```python
from build123d import *

# Parameters (mm, degrees)
AUFSATZ_LINEAR_AUSTRAGEN1_DEPTH      = 25
AUFSATZ_LINEAR_AUSTRAGEN1_DEPTH_BACK = 12.5
SKIZZE1_W                            = 33
SKIZZE1_H                            = 15
SKIZZE2_W                            = 28
SKIZZE2_H                            = 12
SCHNITT_LINEAR_AUSTRAGEN1_DEPTH      = 42.650330131
M3_GEWINDEBOHRUNG1_D                 = 2.5
M4_GEWINDEBOHRUNG1_D                 = 3.3
SCHNITT_LINEAR_AUSTRAGEN2_DEPTH      = 34.5


with BuildPart() as part:
    # Skizze1 → Aufsatz-Linear austragen1 (new, two sides: drawn at the far end of the back side and taken through both)
    with BuildSketch(Plane.XY.offset(-AUFSATZ_LINEAR_AUSTRAGEN1_DEPTH_BACK)):
        Rectangle(SKIZZE1_W, SKIZZE1_H)
    extrude(amount=AUFSATZ_LINEAR_AUSTRAGEN1_DEPTH + AUFSATZ_LINEAR_AUSTRAGEN1_DEPTH_BACK)

    # Skizze2 → Schnitt-Linear austragen1 (cut, through all)
    with BuildSketch(Plane.XY.offset(25)):
        with Locations((-2.5, -1.5)):
            Rectangle(SKIZZE2_W, SKIZZE2_H)
    extrude(amount=-SCHNITT_LINEAR_AUSTRAGEN1_DEPTH, mode=Mode.SUBTRACT)

    # M3 Gewindebohrung1 (through all)
    with Locations(Plane(origin=(0, 7.5, 0), x_dir=(1, 0, 0), z_dir=(0, 1, 0))):
        with Locations((-9.5, 0)):
            Hole(M3_GEWINDEBOHRUNG1_D / 2)

    # M4 Gewindebohrung1 (through all)
    with Locations(Plane(origin=(16.5, 0, 0), x_dir=(0, 0, -1), z_dir=(1, 0, 0))):
        with Locations((-4.25, -0.5), (4.25, -0.5)):
            Hole(M4_GEWINDEBOHRUNG1_D / 2)

    # Skizze7 → Schnitt-Linear austragen2 (cut, through all)
    with BuildSketch(Plane(origin=(0, 7.5, 0), x_dir=(1, 0, 0), z_dir=(0, 1, 0))):
        Polygon((0, -25), (-16.5, -12.5), (-16.5, -25), align=None)
    extrude(amount=-SCHNITT_LINEAR_AUSTRAGEN2_DEPTH, mode=Mode.SUBTRACT)


solid = part.part
```
Geometry check sheet. Reference: the model listing, model coordinates, mm. A direction names the side the tool comes from. Coordinates: 2 decimals unless noted, no trailing zeros. Write each loop counter-clockwise with the first axis right and the second up, starting at its lowest first coordinate (ties: lowest second). Pieces come first, ordered by that corner, then holes. Notation, with made-up numbers: M 69.5,53 L 103.5,53 A27 ccw 103.5,78 Z; hole C 13.25,-21.75 d9. An arc over 180 degrees is marked long. One line per item, written item: value. Start each with the question number.
(1) Sectioned sample at A-A, the plane z = 0. Enter the section's corners in (x, y), and give its area (4 significant figures).
(2) Sectioned sample at D-D, the plane x = -9.5. Enter the section's corners in (y, z).
(3) Scan lines: line 1 along X through (y, z) = (-2.25, 13); line 2 along Y through (x, z) = (5, 19); line 3 along Z through (x, y) = (12.5, -1.75). Record each from-to range of solid material in increasing order. Write a range as [from, to].
(4) Release check for a two-part mould opening along Z. For faces 1 (the face through (-8.13, 6.02, 18.84)), 2 (the face through (-3, 4.5, 7)), 3 (the face through (13.97, -0.43, -5.9)), 4 (the face through (13.97, -0.43, 2.6)) record: released by +Z, released by -Z, zero draft, split by the parting line, or undercut.
(5) Depth check by flat-ended pin: pin 1 (12 mm diameter, centred on x = 5, z = 20.5, fed in from -Y); pin 2 (4.5 mm diameter, centred on y = -0.5, z = 4.25, fed in from -X). Enter the tip coordinate at first touch or a pass-through.
(6) Sectioned sample at B-B, the plane y = -0.5. Enter the section's corners in (x, z), and give its area (4 significant figures).
(7) Tool access check on faces 5 (the face through (12, 2, 25)), 6 (the face through (11.5, -2, 7)). Record the directions out of +Z, -Z, +X, -X, +Y, -Y that give a thin tool (end or side, any length) a straight path to the whole face; none if there is none.
(8) Sectioned sample at C-C, the plane y = 6.5. Enter the section's corners in (x, z), and give its area (3 significant figures).
Filled sheet:
1. outline: M -16.5,4.5 L -10.75,4.5 L -10.75,7.5 L -16.5,7.5 Z; M -8.25,4.5 L 11.5,4.5 L 11.5,-7.5 L 16.5,-7.5 L 16.5,7.5 L -8.25,7.5 Z
1. area: 151.5 mm²
2. outline: M 4.5,-12.5 L 7.5,-12.5 L 7.5,-1.25 L 4.5,-1.25 Z; M 4.5,1.25 L 7.5,1.25 L 7.5,17.8 L 4.5,17.8 Z
3. line 1: [11.5, 16.5]
3. line 2: [4.5, 7.5]
3. line 3: [-12.5, -5.33], [-3.17, 3.17], [5.33, 25]
4. face 1: released by +Z
4. face 2: zero draft
4. face 3: undercut
4. face 4: undercut
5. pin 1: y = 4.5
5. pin 2: x = 11.5
6. outline: M 11.5,-12.5 L 16.5,-12.5 L 16.5,-5.9 L 11.5,-5.9 Z; M 11.5,-2.6 L 16.5,-2.6 L 16.5,2.6 L 11.5,2.6 Z; M 11.5,5.9 L 16.5,5.9 L 16.5,25 L 11.5,25 Z
6. area: 154.5 mm²
7. face 5: +Z, +X, -X, +Y, -Y
7. face 6: +Z, -Z, -X, -Y
8. outline: M -16.5,-12.5 L 16.5,-12.5 L 16.5,25 L 0,25 L -16.5,12.5 Z; hole C -9.5,0 d2.5
8. area: 1,130 mm²
